Check sheet for the modelled part. Datum: model origin and axes. Units: mm. A direction names the side the tool comes from. Round coordinates to 2 decimals unless told otherwise and drop trailing zeros. Loops run counter-clockwise (first coordinate to the right, second up) from the corner with the lowest first, then second, coordinate; pieces in that order, holes last. Notation, with made-up numbers: (-7, -30.5) - (36, -30.5) arc R22 cw to (36, 0.5) - close; hole circle Ø7 at (57, 62.5). An arc over 180 degrees is marked (long way). Put each result on its own line as item: value. Start each with the question number.
Item 1: Gauge pin test, flat ends, axial feed: pin 1 Ø4 at (x, z) = (34, -40.5) entering from -Y; pin 2 Ø1 at (x, z) = (32.5, -26.5) entering from +Y; pin 3 Ø3 at (x, z) = (12.5, 37) entering from -Y; pin 4 Ø10 at (y, z) = (205, -25.5) entering from -X. Record the tip position at first contact, or that the pin passes through.
Item 2: Section check A-A, the plane x = 0. Record the cut outline in (y, z).
Item 3: Section check B-B, the plane y = 69.5. Record the cut outline in (x, z).
Item 4: Tool access check on faces 1 (the cylindrical face through (23.846, 262.413, -7.509)), 2 (the flat face through (-44.823, 22.524, -26.364)). Record the directions out of +Z, -Z, +X, -X, +Y, -Y that give a thin tool (end or side, any length) a straight path to the whole face; none if there is none.
Item 5: Material ranges on line 1 along Y through (x, z) = (0.5, 46.5); line 2 along Z through (x, y) = (-39.5, 34); line 3 along X through (y, z) = (185.5, -15), recorded low to high.
from build123d import *

# Parameters (mm, degrees)
BOSS_EXTRUDE1_DEPTH = 45
SKETCH2_R           = 25
BOSS_EXTRUDE2_DEPTH = 445
CHAMFER1_SIZE       = 4


with BuildPart() as part:
    # Sketch1 → Boss-Extrude1 (new body)
    with BuildSketch(Plane(origin=(0, 0, 0), x_dir=(1, 0, 0), z_dir=(0, 1, 0))):
        Polygon((-60.044427996, 0), (-30.022213998, -52), (30.022213998, -52), (60.044427996, 0), (30.022213998, 52), (-30.022213998, 52), align=None)
    extrude(amount=BOSS_EXTRUDE1_DEPTH)

    # Sketch2 → Boss-Extrude2 (add)
    with BuildSketch(Plane(origin=(0, 45, 0), x_dir=(1, 0, 0), z_dir=(0, 1, 0))):
        Circle(SKETCH2_R)
    extrude(amount=BOSS_EXTRUDE2_DEPTH)

    # Sketch3 → Cut-Revolve1 (revolve, cut)
    with BuildSketch(Plane.XY):
        with BuildLine():
            Line((48.044427996, 0), (60.044427996, 0))
            Line((60.044427996, 0), (60.044427996, 12))
            ThreePointArc((60.044427996, 12), (56.52970937, 3.514718626), (48.044427996, 0))
        make_face()
    revolve(axis=Axis((0, 490, 0), (0, -1, 0)), mode=Mode.SUBTRACT)

    # Chamfer1
    chamfer1_edges = [part.edges().sort_by_distance(p)[0] for p in [
        (-25, 490, 0),
    ]]
    chamfer(chamfer1_edges, length=CHAMFER1_SIZE)


solid = part.part
Check result:
1. pin 1: y = 0.34
1. pin 2: y = 45
1. pin 3: y = 0
1. pin 4: x = -14.31
2. outline: (0, -48.04) arc R12 ccw to (0.67, -52) - (45, -52) - (45, -25) - (486, -25) - (490, -21) - (490, 21) - (486, 25) - (45, 25) - (45, 52) - (0.67, 52) arc R12 ccw to (0, 48.04) - close
3. outline: circle Ø50 at (0, 0)
4. face 1: +Y
4. face 2: -Z, -X, +Y, -Y
5. line 1: 0 to 45
5. line 2: -35.58 to 35.58
5. line 3: -20 to 20
